Here's how the part is built. I have some questions about the finished solid (model axes, mm). A direction names the side the tool comes from. Round coordinates to 2 decimals unless told otherwise and drop trailing zeros. Loops run counter-clockwise (first coordinate to the right, second up) from the corner with the lowest first, then second, coordinate; pieces in that order, holes last. Notation, with made-up numbers: M -28,11.25 L -22,11.25 A28 ccw -22,50.25 Z; hole C -23.75,-22.5 d6. An arc over 180 degrees is marked long. Answer as a JSON object with one key per item and string values.
from build123d import *

# Parameters (mm, degrees)
SWEEP1_PROFILE_R = 6
CHAMFER1_SIZE    = 2


with BuildPart() as part:
    # Sweep1: sweep along a path in Sketch1
    with BuildLine(Plane.XY) as sweep1_path:
        Line((75, 90), (10, 90))
        ThreePointArc((10, 90), (2.928932188, 87.071067812), (0, 80))
        Line((0, 80), (0, 0))
    # Sweep1 profile (on start of the path) → Sweep1 (sweep)
    with BuildSketch(Plane(origin=(75, 90, 0), x_dir=(0, -1, 0), z_dir=(-1, 0, 0))):
        Circle(SWEEP1_PROFILE_R)
    sweep(path=sweep1_path.line)

    # Chamfer1
    chamfer1_edges = [part.edges().sort_by_distance(p)[0] for p in [
        (-6, 0, 0),
        (75, 96, 0),
    ]]
    chamfer(chamfer1_edges, length=CHAMFER1_SIZE)


solid = part.part
Item 1: For P1, Ø4, axis at x = 3, z = 3, coming from the +Y side; P2, Ø3, axis at x = 49.5, z = -4, coming from the -Y side; P3, Ø1.5, axis at x = 32, z = -2, coming from the +Y side, each with a flat end and sliding along its axis, tell me the tip position at first contact or that it passes through.
Solution:
{"P1": "stops at y = 94.77", "P2": "stops at y = 84.55", "P3": "stops at y = 95.87"}
Item 2: I want a section at C-C on x = 35. List the corners of the cut face in (y, z) for me, plus the area to 3 significant figures.
Solution:
{"outline": "C 90,0 d12", "area": "113 mm2"}
Item 3: If I drill on L1, parallel to Y at x = 24.5, z = -0.25; L2, parallel to X at y = 11, z = -5.5; L3, parallel to X at y = 4.5, z = 3.5, over which ranges is the centre line in solid material (lowest first)? Write a range as from..to.
Solution:
{"L1": "y = 84.01..95.99", "L2": "x = -2.4..2.4", "L3": "x = -4.87..4.87"}
Item 4: For faces 1 (the face through (0, 0, 0)), 2 (the face through (41, 96, 0)), 3 (the face through (-6, 40, 0)), which set-ups out of +Z, -Z, +X, -X, +Y, -Y let a thin tool reach every point of the face, with its end or its side?
Solution:
{"face 1": "+Z, -Z, +X, -X, -Y", "face 2": "+X", "face 3": "-Y"}
Item 5: I want a section at A-A on z = 0. List the corners of the cut face in (x, y) for me, plus the area to 3 significant figures.
Solution:
{"outline": "M -6,2 L -4,0 L 4,0 L 6,2 L 6,80 A4 cw 10,84 L 73,84 L 75,86 L 75,94 L 73,96 L 10,96 A16 ccw -6,80 Z", "area": "1,920 mm2"}
Item 6: I want a section at B-B on y = 45.5. List the corners of the cut face in (x, z) for me, plus the area to 3 significant figures.
Solution:
{"outline": "C 0,0 d12", "area": "113 mm2"}
